For this review, take the finished solid that the model builds, in its own axes (mm). Face numbers are marked on the shaded views. A direction names the side the tool comes from. Give positions to 0.01 mm unless a question says otherwise; leave off trailing zeros. Order: outer loops, then holes, each group sorted by start corner. A loop starts at its lowest first (then second) coordinate and runs counter-clockwise, first axis right, second up. Notation, with made-up numbers: (80, -29) - (125, -29) arc R16 cw to (125, -2) - close; hole circle Ø11 at (52.5, 30.25). An arc over 180 degrees is marked (long way). One line per item, written item: value.
```python
from build123d import *

# Parameters (mm, degrees)
F0_W     = 304.8
F0_H     = 50.8
F1_DEPTH = 19.05
F2_W     = 50.8
F2_H     = 152.4
F3_DEPTH = 12.7
F4_R     = 6.35
F5_DEPTH = 12.7


# Not quite as in the source:
# - a pattern or mirror of a feature is missing from the dataset's text; its kind, count and spacing are read off the source's solid


with BuildPart() as f1:
    # F0 (on Top) → F1 (new body)
    with BuildSketch(Plane.XY):
        Rectangle(F0_W, F0_H)
    extrude(amount=F1_DEPTH)

    # F2 (on face) → F3 (join)
    with BuildSketch(Plane.YZ.offset(152.4)):
        with Locations((0, -57.15)):
            Rectangle(F2_W, F2_H)
    f3 = extrude(amount=F3_DEPTH)

    # F3_copies: F3 across plane
    add(f3.mirror(Plane(origin=(0, 0, 0), x_dir=(0, 0, -1), z_dir=(-1, 0, 0))))

    # F4 (on face) → F5 (cut, through all)
    with BuildSketch(Plane.YZ.offset(165.1)):
        with Locations((0, -120.65)):
            Circle(F4_R)
        with Locations((0, -82.55)):
            Circle(F4_R)
    f5 = extrude(amount=-F5_DEPTH, mode=Mode.SUBTRACT)

    # F5_copies: F5 across plane
    add(f5.mirror(Plane(origin=(0, 0, 0), x_dir=(0, 0, -1), z_dir=(-1, 0, 0))), mode=Mode.SUBTRACT)


solid = f1.part
```
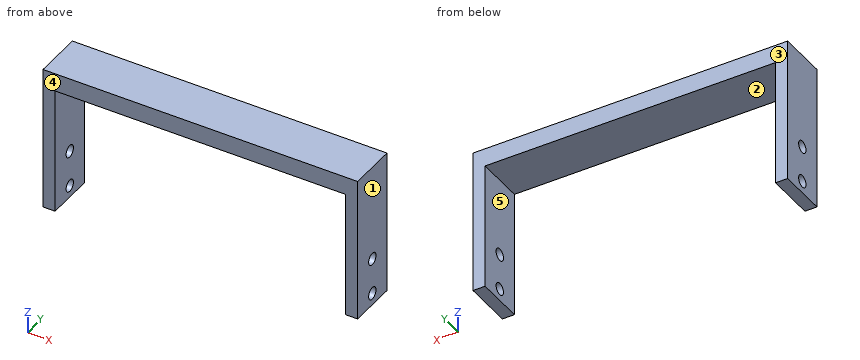
(1) Draft analysis for pull direction X (two halves, no side actions). For the marked faces 1, 2 and 3, state which applies: pulls with the +X half, pulls with the -X half, needs draft (parallel to the pull), parting line crosses it, or undercut.
Answers below:
face 1: pulls with the +X half
face 2: undercut
face 3: needs draft
(2) Machinability: for the marked faces 4 and 5, which of the approach directions +Z, -Z, +X, -X, +Y, -Y give a long, thin tool a straight path to every point of the face, cutting with its end or side? Answer none if there is none.
Answers below:
face 4: +Z, -Z, +X, -X, -Y
face 5: -Z, +Y, -Y
(3) Wall thickness on line 1 (Z direction, x = 156, y = 0); line 2 (X direction, y = 11, z = -126); line 3 (Z direction, x = 124, y = 23): over which ranges is each line inside the solid? List them lowest first. Write a range as from..to.
Answers below:
line 1: z = -133.35..-127, -114.3..-88.9, -76.2..19.05
line 2: x = -165.1..-152.4, 152.4..165.1
line 3: z = 0..19.05
(4) Take a section at A-A (y = 0). Write out the cut boundary in (x, z).
Answers below:
outline: (-165.1, -133.35) - (-152.4, -133.35) - (-152.4, -127) - (-165.1, -127) - close; (-165.1, -114.3) - (-152.4, -114.3) - (-152.4, -88.9) - (-165.1, -88.9) - close; (-165.1, -76.2) - (-152.4, -76.2) - (-152.4, 0) - (152.4, 0) - (152.4, -76.2) - (165.1, -76.2) - (165.1, 19.05) - (-165.1, 19.05) - close; (152.4, -133.35) - (165.1, -133.35) - (165.1, -127) - (152.4, -127) - close; (152.4, -114.3) - (165.1, -114.3) - (165.1, -88.9) - (152.4, -88.9) - close
(5) Take a section at D-D (y = 18). Write out the cut boundary in (x, z), then the cut area to 3 significant figures.
Answers below:
outline: (-165.1, -133.35) - (-152.4, -133.35) - (-152.4, 0) - (152.4, 0) - (152.4, -133.35) - (165.1, -133.35) - (165.1, 19.05) - (-165.1, 19.05) - close
area: 9,680 mm^2
(6) Take a section at C-C (z = -25.5). Write out the cut boundary in (x, y).
Answers below:
outline: (-165.1, -25.4) - (-152.4, -25.4) - (-152.4, 25.4) - (-165.1, 25.4) - close; (152.4, -25.4) - (165.1, -25.4) - (165.1, 25.4) - (152.4, 25.4) - close
(7) Take a section at B-B (z = -82.55). Write out the cut boundary in (x, y), then the cut area to 3 significant figures.
Answers below:
outline: (-165.1, -25.4) - (-152.4, -25.4) - (-152.4, -6.35) - (-165.1, -6.35) - close; (-165.1, 6.35) - (-152.4, 6.35) - (-152.4, 25.4) - (-165.1, 25.4) - close; (152.4, -25.4) - (165.1, -25.4) - (165.1, -6.35) - (152.4, -6.35) - close; (152.4, 6.35) - (165.1, 6.35) - (165.1, 25.4) - (152.4, 25.4) - close
area: 968 mm^2
(8) For P1, Ø5, axis at x = 32, y = -18.5, coming from the -Z side; P2, Ø7.5, axis at y = 0, z = -120.65, coming from the +X side, all flat-tipped, find the tip position at first contact; note any pin that passes through.
Answers below:
P1: stops at z = 0
P2: passes through
